Source: CAD feature listing. Evaluate the final solid. Frame: model axes, mm. Face numbers are marked on the shaded views. A direction names the side the tool comes from. Give positions to 0.01 mm unless a question says otherwise; leave off trailing zeros. Order: outer loops, then holes, each group sorted by start corner. A loop starts at its lowest first (then second) coordinate and runs counter-clockwise, first axis right, second up. Notation, with made-up numbers: (64.5, -10) -> (95.5, -10) arc R28 ccw to (95.5, 23) -> close; hole circle Ø2 at (54, 48.5). An arc over 180 degrees is marked (long way). Use one line per item in the form item = value. Start each with the question number.
from build123d import *

# Parameters (mm, degrees)
SKETCH1_R           = 3.683
SKETCH1_R_2         = 1.143
BOSS_EXTRUDE1_DEPTH = 1.27
FILLET1_R           = 6.35
BOSS_EXTRUDE2_DEPTH = 7.239
FILLET2_R           = 1.27


with BuildPart() as part:
    # Sketch1 → Boss-Extrude1 (new body)
    with BuildSketch(Plane(origin=(0, 0, 0), x_dir=(1, 0, 0), z_dir=(0, 1, 0))):
        with BuildLine():
            ThreePointArc((-7.094482759, 2.780775861), (-10.16, 0), (-7.094482759, -2.780775861))
            ThreePointArc((-7.094482759, -2.780775861), (0, -7.62), (7.094482759, -2.780775861))
            ThreePointArc((7.094482759, -2.780775861), (10.16, 0), (7.094482759, 2.780775861))
            ThreePointArc((7.094482759, 2.780775861), (0, 7.62), (-7.094482759, 2.780775861))
        make_face()
        Circle(SKETCH1_R, mode=Mode.SUBTRACT)
        with Locations((7.366, 0)):
            Circle(SKETCH1_R_2, mode=Mode.SUBTRACT)
        with Locations((-7.366, 0)):
            Circle(SKETCH1_R_2, mode=Mode.SUBTRACT)
    extrude(amount=BOSS_EXTRUDE1_DEPTH)

    # Fillet1
    fillet1_edges = [part.edges().sort_by_distance(p)[0] for p in [
        (7.094482759, 0.635, -2.780775861),
        (7.094482759, 0.635, 2.780775861),
        (-7.094482759, 0.635, 2.780775861),
        (-7.094482759, 0.635, -2.780775861),
    ]]
    fillet(fillet1_edges, radius=FILLET1_R)

    # Sketch2 → Boss-Extrude2 (add)
    with BuildSketch(Plane(origin=(0, 1.27, 0), x_dir=(1, 0, 0), z_dir=(0, 1, 0))):
        with BuildLine():
            Line((-6.148361062, -1.5875), (-7.452801067, -1.5875))
            ThreePointArc((-7.452801067, -1.5875), (-6.951653953, -3.120722244), (-6.138996865, -4.514102069))
            ThreePointArc((-6.138996865, -4.514102069), (0, -7.62), (6.138996865, -4.514102069))
            ThreePointArc((6.138996865, -4.514102069), (6.951653953, -3.120722244), (7.452801067, -1.5875))
            Line((7.452801067, -1.5875), (6.148361062, -1.5875))
            ThreePointArc((6.148361062, -1.5875), (0, -6.35), (-6.148361062, -1.5875))
        make_face()
        with BuildLine():
            ThreePointArc((6.148361062, 1.5875), (0, 6.35), (-6.148361062, 1.5875))
            Line((-6.148361062, 1.5875), (-7.452801067, 1.5875))
            ThreePointArc((-7.452801067, 1.5875), (0, 7.62), (7.452801067, 1.5875))
            Line((7.452801067, 1.5875), (6.148361062, 1.5875))
        make_face()
    extrude(amount=BOSS_EXTRUDE2_DEPTH)

    # Fillet2
    fillet2_edges = [part.edges().sort_by_distance(p)[0] for p in [
        (-6.800581065, 8.509, 1.5875),
        (6.800581065, 8.509, 1.5875),
        (6.800581065, 8.509, -1.5875),
        (-6.800581065, 8.509, -1.5875),
    ]]
    fillet(fillet2_edges, radius=FILLET2_R)


solid = part.part
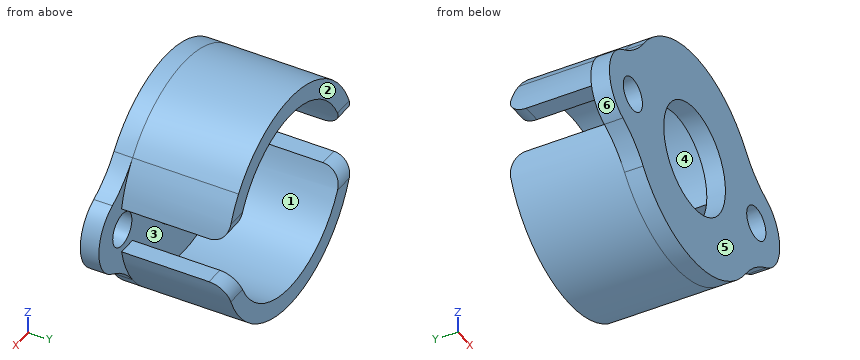
1) Reachability of the marked faces 1 and 2 from +Z, -Z, +X, -X, +Y, -Y: full face, straight path, thin tool, end or side. Return the list, or none.
2) Cut plane A-A, the plane y = 5.25. Return the cut outline in (x, z), plus the area to 3 significant figures.
3) Material intervals for probe 1 along Z at (x, y) = (0, 0.45); probe 2 along Z at (x, y) = (-0.25, 4.75); probe 3 along Y at (x, z) = (-2.75, 5.5), sorted ascending.
4) Draft query along Z for the marked faces 3, 4, 5 and 6. Return one class per face: +Z half, -Z half, draft (parallel to the pull), parting line (faces both ways), or undercut.
5) Pin query (flat end, axial travel): pin 1 (0.7 mm diameter, centred on x = 7, y = 4, fed in from +Z); pin 2 (4 mm diameter, centred on x = -6.5, y = 7.5, fed in from +Z); pin 3 (1.8 mm diameter, centred on x = -7.366, z = 0, fed in from -Y); pin 4 (1 mm diameter, centred on x = -7, y = 3, fed in from -Z). Return the tip coordinate at first contact, or that it passes through.
6) Cut plane C-C, the plane x = -4.5. Return the cut outline in (y, z), plus the area to 3 significant figures.
7) Cut plane B-B, the plane x = 0. Return the cut outline in (y, z).
Output values:
q1.face_1 = +Y
q1.face_2 = +Z, -Z, +X, -X, +Y
q2.outline = (-7.45, -1.59) arc R7.62 ccw to (7.45, -1.59) -> (6.15, -1.59) arc R6.35 cw to (-6.15, -1.59) -> close; (-7.45, 1.59) -> (-6.15, 1.59) arc R6.35 cw to (6.15, 1.59) -> (7.45, 1.59) arc R7.62 ccw to start
q2.area = 47.6 mm^2
q3.probe_1 = -7.62 to -3.68, 3.68 to 7.62
q3.probe_2 = -7.62 to -6.35, 6.35 to 7.62
q3.probe_3 = 0 to 1.27
q4.face_3 = undercut
q4.face_4 = undercut
q4.face_5 = draft
q4.face_6 = parting line
q5.pin_1 = 3.72
q5.pin_2 = 6.15
q5.pin_3 = through
q5.pin_4 = -3.98
q6.outline = (0, -6.15) -> (8.51, -6.15) -> (8.51, -4.48) -> (1.27, -4.48) -> (1.27, 4.48) -> (8.51, 4.48) -> (8.51, 6.15) -> (0, 6.15) -> close
q6.area = 39.8 mm^2
q7.outline = (0, -7.62) -> (8.51, -7.62) -> (8.51, -6.35) -> (1.27, -6.35) -> (1.27, -3.68) -> (0, -3.68) -> close; (0, 3.68) -> (1.27, 3.68) -> (1.27, 6.35) -> (8.51, 6.35) -> (8.51, 7.62) -> (0, 7.62) -> close
